Design review of the part built by this model. Coordinates are the model's own, in mm. A direction names the side the tool comes from. Give positions to 0.01 mm unless a question says otherwise; leave off trailing zeros. Loops run counter-clockwise (first coordinate to the right, second up) from the corner with the lowest first, then second, coordinate; pieces in that order, holes last. Notation, with made-up numbers: M -13.5,-37.5 L 40.5,-37.5 A11 cw 40.5,-23.5 Z; hole C 80,57 d5. An arc over 180 degrees is marked long. Use a Markdown table: item, result. Add a question column.
(1) For probe 1 along X at (y, z) = (7, 11); probe 2 along Z at (x, y) = (8, -5.25); probe 3 along Z at (x, y) = (-8, -6.25), list the stretches that pass through material, from the lowest coordinate up.
(2) Add section C-C, the plane y = 8.75. Give the boundary of the cut face in (x, z), then the cut area to 3 significant figures.
(3) Draft analysis for pull direction X (two halves, no side actions). For faces 1 (the face through (-3.37, -6.48, 10.71)), 2 (the face through (4.12, -6.52, -7.83)), 3 (the face through (-9, 2, -3)), 4 (the face through (7, -8, -7)), state which applies: pulls with the +X half, pulls with the -X half, needs draft (parallel to the pull), parting line crosses it, or undercut.
(4) Add section D-D, the plane y = -1. Give the boundary of the cut face in (x, z).
(5) For faces 5 (the face through (-6.234, -6.521, 10.031)), 6 (the face through (-6.97, -2.46, 7.24)), 7 (the face through (-4.12, -6.52, 7.83)), 8 (the face through (5, -5, -9)), list the 3-axis set-ups (+Z, -Z, +X, -X, +Y, -Y) from which the entire face can be reached by the end or side of a thin tool; tool diameter is ignored.
(6) Insertion check: pin 1 Ø1.5 at (x, z) = (9.5, 6) entering from -Y; pin 2 Ø3 at (x, y) = (-12, 9) entering from +Z; pin 3 Ø1.5 at (x, y) = (9.5, 2.5) entering from -Z; pin 4 Ø4.5 at (x, z) = (8, -13.86) entering from -Y. Each pin has a flat end and moves straight along its axis. Give the tip position at first contact, or say it passes through.
(7) Add section B-B, the plane z = 0. Give the boundary of the cut face in (x, y).
(8) Add section A-A, the plane x = 0. Give the boundary of the cut face in (y, z).
```python
from build123d import *

# Parameters (mm, degrees)
ESQUISSE1_R                                 = 22.5
BOSS_EXTRU_1_DEPTH                          = 4
ESQUISSE2_R                                 = 4
BOSS_EXTRU_3_DEPTH                          = 8.5
CHANFREIN1_SIZE                             = 8.5
CHANFREIN1_SIZE_2                           = 0.445466124
ESQUISSE4_R                                 = 2.554533876
ENL_V_MAT_EXTRU_1_DEPTH                     = 35.186985828
R_P_TITION_CIRCULAIRE1_COUNT                = 3
CHANFREIN1_OF_R_P_TITION_CIRCULAIRE1_SIZE   = 8.5
CHANFREIN1_OF_R_P_TITION_CIRCULAIRE1_SIZE_2 = 0.445466124
ENL_V_MAT_EXTRU_2_REACH                     = 34.936
ESQUISSE5_R                                 = 8.5
ENL_V_START                                 = -4
ESQUISSE6_W                                 = 22
ESQUISSE6_H                                 = 6
ENL_V_MAT_EXTRU_4_DEPTH                     = 4
BOSS_EXTRU_5_DEPTH                          = 8
ESQUISSE8_W                                 = 3.05
ESQUISSE8_H                                 = 3
BOSS_EXTRU_6_DEPTH                          = 5
R_P_TITION_CIRCULAIRE3_COUNT                = 2


with BuildPart() as part:
    # Esquisse1 → Boss.-Extru.1 (new body)
    with BuildSketch(Plane(origin=(0, 0, 0), x_dir=(1, 0, 0), z_dir=(0, 1, 0))):
        with Locations(Location((0, 0, 0), (0, 0, 270))):
            Circle(ESQUISSE1_R)
    extrude(amount=BOSS_EXTRU_1_DEPTH)

    # Esquisse2 → Boss.-Extru.3 (add)
    with BuildSketch(Plane(origin=(0, 4, 0), x_dir=(1, 0, 0), z_dir=(0, 1, 0))):
        with Locations(Location((-16, 0, 0), (0, 0, 270))):
            Circle(ESQUISSE2_R)
    boss_extru_3 = extrude(amount=BOSS_EXTRU_3_DEPTH)

    # Chanfrein1
    # the kernel refuses this chamfer: 8.5, 0.445466124 mm, written as the material it takes off along each edge
    with BuildSketch(Plane(origin=(-16, 12.5, 0), x_dir=(0, 0, 1), z_dir=(-1, 0, 0))) as chanfrein1_piece_1_section:
        Polygon((4, -CHANFREIN1_SIZE), (4 - CHANFREIN1_SIZE_2, 0), (4, 0), align=None)
    chanfrein1_piece_1 = revolve(axis=Axis((-16, 12.5, 0), (0, 1, 0)), mode=Mode.PRIVATE)
    chanfrein1_piece_1 = split(chanfrein1_piece_1, bisect_by=Plane(origin=(-16, 4, -3.812448858), z_dir=(0, 1, 0)), keep=Keep.TOP, mode=Mode.PRIVATE)
    add(chanfrein1_piece_1, mode=Mode.SUBTRACT)

    # Esquisse4 → Enlèv. mat.-Extru.1 (cut, through all)
    with BuildSketch(Plane(origin=(0, 12.5, 0), x_dir=(1, 0, 0), z_dir=(0, 1, 0))):
        with Locations(Location((-16, 0, 0), (0, 0, 270))):
            Circle(ESQUISSE4_R)
    enl_v_mat_extru_1 = extrude(amount=-ENL_V_MAT_EXTRU_1_DEPTH, mode=Mode.SUBTRACT)

    # Répétition circulaire1: Boss.-Extru.3, Enlèv. mat.-Extru.1 ×3 about axis
    r_p_tition_circulaire1_axis = Axis((0, 0, 0), (0, 1, 0))
    add([boss_extru_3.rotate(r_p_tition_circulaire1_axis, i * 360 / R_P_TITION_CIRCULAIRE1_COUNT) for i in range(1, R_P_TITION_CIRCULAIRE1_COUNT)])
    add([enl_v_mat_extru_1.rotate(r_p_tition_circulaire1_axis, i * 360 / R_P_TITION_CIRCULAIRE1_COUNT) for i in range(1, R_P_TITION_CIRCULAIRE1_COUNT)], mode=Mode.SUBTRACT)

    # Chanfrein1 of Répétition circulaire1
    # the kernel refuses this chamfer: 8.5, 0.445466124 mm, written as the material it takes off along each edge
    with BuildSketch(Plane(origin=(8, 12.5, 13.856406461), x_dir=(0.8660254037844387, 0, -0.5000000000000001), z_dir=(0.5000000000000001, 0, 0.8660254037844387))) as chanfrein1_of_r_p_tition_circulaire1_piece_1_section:
        Polygon((4, -CHANFREIN1_OF_R_P_TITION_CIRCULAIRE1_SIZE), (4 - CHANFREIN1_OF_R_P_TITION_CIRCULAIRE1_SIZE_2, 0), (4, 0), align=None)
    chanfrein1_of_r_p_tition_circulaire1_piece_1 = revolve(axis=Axis((8, 12.5, 13.856406461), (0, 1, 0)), mode=Mode.PRIVATE)
    chanfrein1_of_r_p_tition_circulaire1_piece_1 = split(chanfrein1_of_r_p_tition_circulaire1_piece_1, bisect_by=Plane(origin=(4.698322438, 4, 15.762630889), z_dir=(0, 1, 0)), keep=Keep.TOP, mode=Mode.PRIVATE)
    add(chanfrein1_of_r_p_tition_circulaire1_piece_1, mode=Mode.SUBTRACT)
    with BuildSketch(Plane(origin=(8, 12.5, -13.856406461), x_dir=(-0.8660254037844384, 0, -0.5000000000000003), z_dir=(0.5000000000000003, 0, -0.8660254037844384))) as chanfrein1_of_r_p_tition_circulaire1_piece_2_section:
        Polygon((4, -CHANFREIN1_OF_R_P_TITION_CIRCULAIRE1_SIZE), (4 - CHANFREIN1_OF_R_P_TITION_CIRCULAIRE1_SIZE_2, 0), (4, 0), align=None)
    chanfrein1_of_r_p_tition_circulaire1_piece_2 = revolve(axis=Axis((8, 12.5, -13.856406461), (0, 1, 0)), mode=Mode.PRIVATE)
    chanfrein1_of_r_p_tition_circulaire1_piece_2 = split(chanfrein1_of_r_p_tition_circulaire1_piece_2, bisect_by=Plane(origin=(11.301677562, 4, -11.950182032), z_dir=(0, 1, 0)), keep=Keep.TOP, mode=Mode.PRIVATE)
    add(chanfrein1_of_r_p_tition_circulaire1_piece_2, mode=Mode.SUBTRACT)

    # Esquisse5 → Enlèv. mat.-Extru.2 (cut, up to next)
    with BuildSketch(Plane(origin=(0, 4, 0), x_dir=(1, 0, 0), z_dir=(0, 1, 0)), mode=Mode.PRIVATE) as enl_v_mat_extru_2_sk1:
        with Locations(Location((0, 0, 0), (0, 0, 270))):
            Circle(ESQUISSE5_R)
    enl_v_mat_extru_2_tool1 = extrude(enl_v_mat_extru_2_sk1.sketch, amount=-ENL_V_MAT_EXTRU_2_REACH, mode=Mode.PRIVATE) & part.part
    add(enl_v_mat_extru_2_tool1.solids().sort_by_distance((0, 4, 0))[0], mode=Mode.SUBTRACT)

    # Esquisse6 → Enlèv. mat.-Extru.4 (cut)
    with BuildSketch(Plane(origin=(0, 4, 0), x_dir=(1, 0, 0), z_dir=(0, 1, 0)).offset(ENL_V_START)):
        Rectangle(ESQUISSE6_W, ESQUISSE6_H)
    extrude(amount=ENL_V_MAT_EXTRU_4_DEPTH, mode=Mode.SUBTRACT)

    # Esquisse7 → Boss.-Extru.5 (add)
    with BuildSketch(Plane(origin=(0, 0, 0), x_dir=(1, 0, 0), z_dir=(0, 1, 0))):
        with BuildLine():
            Line((-7.95298686, -3), (-11, -3))
            ThreePointArc((-11, -3), (-10.201314207, -6.051828113), (-8.010041275, -8.321162104))
            Line((-8.010041275, -8.321162104), (-5.894835571, -6.123798951))
            ThreePointArc((-5.894835571, -6.123798951), (-7.097892398, -4.676529002), (-7.95298686, -3))
        make_face()
    boss_extru_5 = extrude(amount=-BOSS_EXTRU_5_DEPTH)

    # Esquisse8 → Boss.-Extru.6 (add)
    with BuildSketch(Plane(origin=(0, 0, 0), x_dir=(0.6935100671316063, 0, -0.7204469354415458), z_dir=(0.7204469354415458, 0, 0.6935100671316063))):
        with Locations((-10.025, -6.5)):
            Rectangle(ESQUISSE8_W, ESQUISSE8_H)
    boss_extru_6 = extrude(amount=BOSS_EXTRU_6_DEPTH)

    # Répétition circulaire3: Boss.-Extru.5, Boss.-Extru.6 ×2 about axis
    r_p_tition_circulaire3_axis = Axis((0, 0, 0), (0, 1, 0))
    add([boss_extru_5.rotate(r_p_tition_circulaire3_axis, i * 360 / R_P_TITION_CIRCULAIRE3_COUNT) for i in range(1, R_P_TITION_CIRCULAIRE3_COUNT)])
    add([boss_extru_6.rotate(r_p_tition_circulaire3_axis, i * 360 / R_P_TITION_CIRCULAIRE3_COUNT) for i in range(1, R_P_TITION_CIRCULAIRE3_COUNT)])


solid = part.part
```
Established:
| question | item | result |
|---|---|---|
| 1 | probe 1 | 5.43 to 10.57 |
| 1 | probe 2 | -8.33 to -3 |
| 1 | probe 3 | 3 to 8.33 |
| 2 | outline | C -16,0 d7.5; C 8,-13.86 d7.5; C 8,13.86 d7.5; hole C -16,0 d5.11; hole C 8,-13.86 d5.11; hole C 8,13.86 d5.11 |
| 2 | area | 71.1 mm^2 |
| 3 | face 1 | pulls with the +X half |
| 3 | face 2 | pulls with the -X half |
| 3 | face 3 | undercut |
| 3 | face 4 | needs draft |
| 4 | outline | M -11,3 L -7.95,3 A8.5 cw -5.89,6.12 L -8.01,8.32 A6.23 ccw Z; M 5.89,-6.12 L 8.01,-8.32 A6.23 ccw 11,-3 L 7.95,-3 A8.5 cw Z |
| 5 | face 5 | +Z, -X, -Y |
| 5 | face 6 | +Z, +X |
| 5 | face 7 | -Z, +X, -Y |
| 5 | face 8 | -Z, -X |
| 6 | pin 1 | y = 0 |
| 6 | pin 2 | z = 2.78 |
| 6 | pin 3 | z = -20.73 |
| 6 | pin 4 | through |
| 7 | outline | M -22.5,0 L -18.55,0 L -18.55,12.5 L -19.55,12.5 L -20,4 L -22.5,4 Z; M -13.45,0 L -11,0 L -11,4 L -12,4 L -12.45,12.5 L -13.45,12.5 Z; M 11,0 L 22.5,0 L 22.5,4 L 11,4 Z |
| 8 | outline | M 0,-22.5 L 4,-22.5 L 4,-8.5 L 0,-8.5 Z; M 0,8.5 L 4,8.5 L 4,22.5 L 0,22.5 Z |
